Part print with two shaded views. Sizes in mm from the minimum x, y, z corner. Give positions to 0.01 mm unless a question says otherwise; leave off trailing zeros. Write each loop counter-clockwise with the first axis right and the second up, starting at its lowest first coordinate (ties: lowest second). Pieces come first, ordered by that corner, then holes. Notation, with made-up numbers: (-24, -17) - (27, -17) arc R14 cw to (27, -10) - close; hole circle Ø4 at (32, -31). An arc over 180 degrees is marked (long way). One line per item, written item: value. Start each with the question number.
(1) Mould opens along Z. For the marked faces 1 and 2 say: pulls with the +Z half, pulls with the -Z half, needs draft (parallel to the pull), parting line crosses it, or undercut.
(2) Cut at A-A, the plane x = 158.5. List the corners of the cut face in (y, z).
(3) Cut at B-B, the plane z = 150. List the corners of the cut face in (x, y).
(4) Drop flat-ended pins along their axis: P1, Ø2.5, axis at x = 190, y = 77, coming from the -Z side; P2, Ø6, axis at y = 47.5, z = 177.5, coming from the +X side; P3, Ø2.5, axis at x = 183, y = 70, coming from the +Z side; P4, Ø1.5, axis at x = 1, y = 34, coming from the -Z side. Give the stop position or say it passes through.
(5) Cut at C-C, the plane y = 43. List the corners of the cut face in (x, z).
(6) Probe L1, parallel to Y at x = 190, z = 231.3; L2, parallel to X at y = 70, z = 231.7; L3, parallel to Z at x = 108.5, y = 66. List the from-to ranges inside material, lowest first.
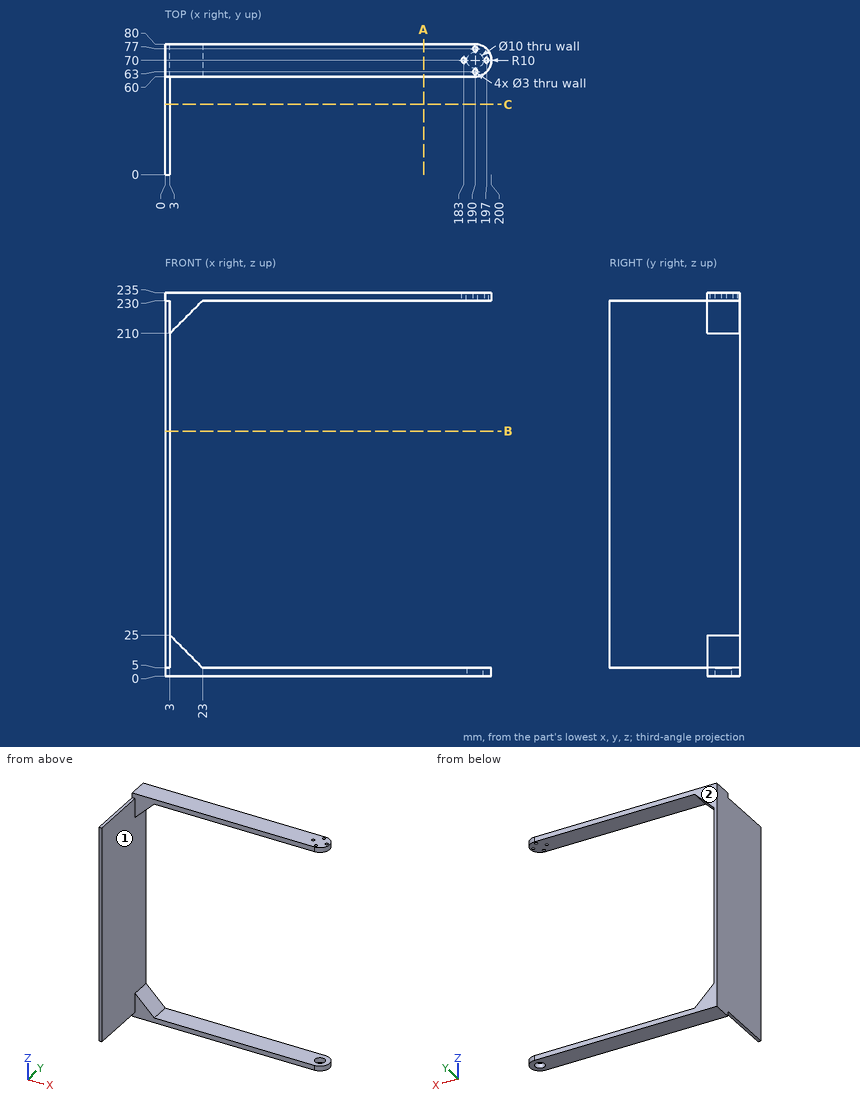
Answers follow:
1. face 1: undercut
1. face 2: needs draft
2. outline: (60, 0) - (80, 0) - (80, 5) - (60, 5) - close; (60, 230) - (80, 230) - (80, 235) - (60, 235) - close
3. outline: (0, 0) - (3, 0) - (3, 80) - (0, 80) - close
4. P1: stops at z = 0
4. P2: stops at x = 3
4. P3: stops at z = 5
4. P4: stops at z = 5
5. outline: (0, 5) - (3, 5) - (3, 230) - (0, 230) - close
6. L1: y = 60 to 61.5, 64.5 to 75.5, 78.5 to 80
6. L2: x = 0 to 181.5, 184.5 to 195.5, 198.5 to 200
6. L3: z = 0 to 5, 230 to 235
